Check sheet for the modelled part. Datum: model origin and axes. Units: mm. Face numbers are marked on the shaded views. A direction names the side the tool comes from. Round coordinates to 2 decimals unless told otherwise and drop trailing zeros. Loops run counter-clockwise (first coordinate to the right, second up) from the corner with the lowest first, then second, coordinate; pieces in that order, holes last. Notation, with made-up numbers: M 61.5,-31.75 L 90.5,-31.75 A14 cw 90.5,-13.75 Z; hole C -37,80 d1. An arc over 180 degrees is marked long. Write item = value, one per line. Start each with the question number.
(1) Go/stop test with a flat-tipped pin: P1, Ø1, axis at x = 26.5, z = 3.5, coming from the +Y side. Record where the tip stops, or that it passes through.
(2) Cross-section at B-B on y = 15.5. Record the boundary of the cut face in (x, z), plus the area to 3 significant figures.
(3) Cross-section at A-A on x = 12. Record the boundary of the cut face in (y, z).
(4) Cross-section at C-C on x = 1. Record the boundary of the cut face in (y, z).
(5) Scan lines: L1, parallel to Y at x = 8, z = 3.35; L2, parallel to X at y = 29.5, z = 0.65; L3, parallel to X at y = 29.5, z = 5.1. Record each from-to range of solid material in increasing order. Write a range as from..to.
(6) Set-up check for the marked faces 1 and 2: record each of +Z, -Z, +X, -X, +Y, -Y from which the full face is reachable in a straight line by a thin tool's end or side.
from build123d import *

# Parameters (mm, degrees)
ESQUISSE1_W             = 38
ESQUISSE1_H             = 34
BOSS_EXTRU_1_DEPTH      = 6
CONG_2_R                = 2
ESQUISSE2_R             = 0.6
BOSS_EXTRU_2_DEPTH      = 3
BOSS_EXTRU_2_DEPTH_BACK = 6


with BuildPart() as part:
    # Esquisse1 → Boss.-Extru.1 (new body)
    with BuildSketch(Plane.XY):
        with Locations((19, 17)):
            Rectangle(ESQUISSE1_W, ESQUISSE1_H)
    extrude(amount=BOSS_EXTRU_1_DEPTH)

    # Congé2
    cong_2_edges = [part.edges().sort_by_distance(p)[0] for p in [
        (38, 17, 6),
        (19, 34, 6),
        (0, 17, 6),
        (19, 34, 0),
        (38, 17, 0),
        (19, 0, 0),
        (0, 17, 0),
        (0, 34, 3),
        (38, 34, 3),
        (38, 0, 3),
        (0, 0, 3),
        (19, 0, 6),
    ]]
    fillet(cong_2_edges, radius=CONG_2_R)

    # Esquisse2 → Boss.-Extru.2 (add, two sides)
    with BuildSketch(Plane(origin=(0, 34, 0), x_dir=(1, 0, 0), z_dir=(0, 1, 0))) as boss_extru_2_sk:
        with Locations((1, -2)):
            Circle(ESQUISSE2_R)
        with Locations((1, -4)):
            Circle(ESQUISSE2_R)
    extrude(amount=BOSS_EXTRU_2_DEPTH)
    extrude(boss_extru_2_sk.sketch, amount=-BOSS_EXTRU_2_DEPTH_BACK)


solid = part.part
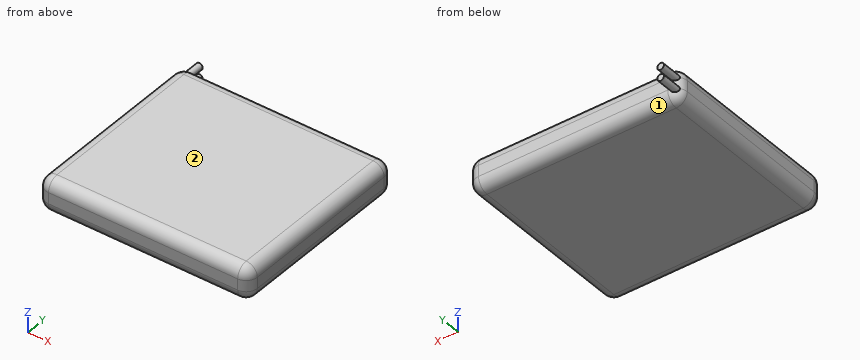
Result:
q1.P1 = 34
q2.outline = M 0,2 A2 ccw 2,0 L 36,0 A2 ccw 38,2 L 38,4 A2 ccw 36,6 L 2,6 A2 ccw 0,4 Z
q2.area = 225 mm^2
q3.outline = M 0,2 A2 ccw 2,0 L 32,0 A2 ccw 34,2 L 34,4 A2 ccw 32,6 L 2,6 A2 ccw 0,4 Z
q4.outline = M 0.27,2 A1.73 ccw 2,0.27 L 32,0.27 A1.73 ccw 33.62,1.4 L 37,1.4 L 37,2.6 L 33.73,2.6 L 33.73,3.4 L 37,3.4 L 37,4.6 L 33.62,4.6 A1.73 ccw 32,5.73 L 2,5.73 A1.73 ccw 0.27,4 Z
q5.L1 = 0..34
q5.L2 = 0.52..37.48
q5.L3 = 0.33..37.67
q6.face_1 = -Z, +X, +Y
q6.face_2 = +Z, +X, -X, +Y, -Y
